from build123d import *

# Parameters (mm, degrees)
SKETCH1_W                                         = 292.1
SKETCH1_H                                         = 6.35
CSK_FOR_4_FLAT_HEAD_MACHINE_SCREW_100_D           = 2.77876
CSK_FOR_4_FLAT_HEAD_MACHINE_SCREW_100_CSINK_D     = 5.715
CSK_FOR_4_FLAT_HEAD_MACHINE_SCREW_100_CSINK_ANGLE = 82


with BuildPart() as part:
    # Sketch1 → Revolve1 (revolve)
    with BuildSketch(Plane.XY, mode=Mode.PRIVATE) as revolve1_sk:
        with Locations((146.05, 3.175)):
            Rectangle(SKETCH1_W, SKETCH1_H)
    revolve(revolve1_sk.sketch.rotate(Axis((292.1, 0, 0), (-1, 0, 0)), 90), axis=Axis((292.1, 0, 0), (-1, 0, 0)))

    # CSK for _4 Flat Head Machine Screw _100 (through all)
    with Locations(Plane.XY.offset(6.35)):
        with Locations((31.75, 0), (260.35, 0)):
            CounterSinkHole(CSK_FOR_4_FLAT_HEAD_MACHINE_SCREW_100_D / 2, CSK_FOR_4_FLAT_HEAD_MACHINE_SCREW_100_CSINK_D / 2, counter_sink_angle=CSK_FOR_4_FLAT_HEAD_MACHINE_SCREW_100_CSINK_ANGLE)


solid = part.part
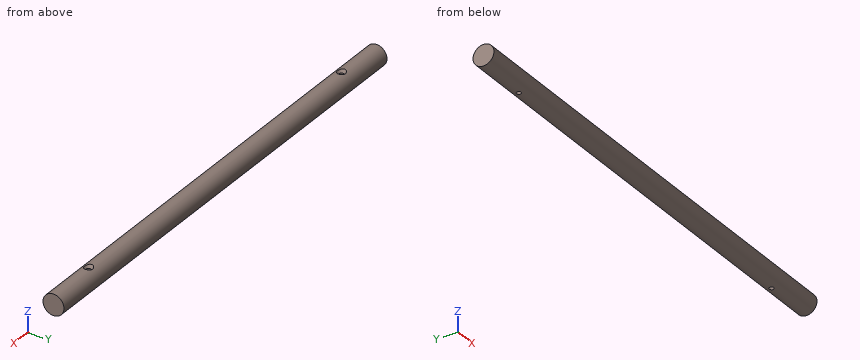
The listing builds one solid part. Answer for the finished solid, in the listing's coordinates (mm). Give positions to 0.01 mm unless a question says otherwise; leave off trailing zeros. Order: outer loops, then holes, each group sorted by start corner. A loop starts at its lowest first (then second) coordinate and runs counter-clockwise, first axis right, second up. Notation, with made-up numbers: (19, 50.25) - (37, 50.25) arc R17 cw to (37, 70.25) - close; hole circle Ø3 at (-6, 76). An arc over 180 degrees is marked (long way). Use one line per item in the form item = value.
1) Find section B-B on x = 184. Determine the outline of the cut face in (y, z).
Verdict:
outline = circle Ø12.7 at (0, 0)
2) Each of these flat-tipped pins is pushed along its axis until it touches: pin 1 (3.5 mm diameter, centred on x = 31.75, y = 0, fed in from +Z); pin 2 (5 mm diameter, centred on x = 258.5, z = 1, fed in from +Y); pin 3 (1.7 mm diameter, centred on x = 260.35, y = 0, fed in from +Z). Where does it stop, or does it pass through?
Verdict:
pin_1 = 5.08
pin_2 = 6.35
pin_3 = through
3) Consider probe 1 along X at (y, z) = (0, -0.25); probe 2 along Y at (x, z) = (31.75, -0.5); probe 3 along X at (y, z) = (0, 5.5). Determine where each line is inside the solid, lowest interval first. Write a range as [from, to].
Verdict:
probe_1 = [0, 30.36], [33.14, 258.96], [261.74, 292.1]
probe_2 = [-6.33, -1.39], [1.39, 6.33]
probe_3 = [0, 29.63], [33.87, 258.23], [262.47, 292.1]
4) Find section A-A on z = -2.75. Determine the outline of the cut face in (x, y), and give its area (3 significant figures).
Verdict:
outline = (0, -5.72) - (292.1, -5.72) - (292.1, 5.72) - (0, 5.72) - close; hole circle Ø2.78 at (31.75, 0); hole circle Ø2.78 at (260.35, 0)
area = 3,330 mm^2
